Here's how the part is built. I have some questions about the finished solid (model axes, mm). Face numbers are marked on the shaded views. Round coordinates to 2 decimals unless told otherwise and drop trailing zeros. Loops run counter-clockwise (first coordinate to the right, second up) from the corner with the lowest first, then second, coordinate; pieces in that order, holes last. Notation, with made-up numbers: (-0.75, 53.25) - (32.25, 53.25) arc R21 cw to (32.25, 62.25) - close; hole circle Ø4 at (-31.75, -39). An arc over 180 degrees is marked (long way). Answer as a JSON object with one key per item and string values. Group by question number.
1) I want a section at A-A, the plane x = -1. Please give me the cut outline in (y, z) (3 decimals).
2) I want a section at B-B, the plane z = 7.5. Please give me the cut outline in (x, y), then the cut area to 3 significant figures.
3) Will these pins go through, and if not, where does the flat tip stop? P1, Ø4, axis at x = 4.5, z = 3, coming from the -Y side; P2, Ø2, axis at x = -1, y = 13, coming from the -Z side; P3, Ø2, axis at y = 12.5, z = 2.5, coming from the -X side; P4, Ø2.5, axis at x = 0, y = 14.15, coming from the +Z side.
4) If we mould it in two halves opening along X, with no side actions, what happens to the marked faces 1, 2 and 3? For each: pulls with the +X half, pulls with the -X half, needs draft (parallel to the pull), parting line crosses it, or undercut.
5) I want a section at C-C, the plane x = -12. Please give me the cut outline in (y, z) (3 decimals), then the cut area to 3 significant figures.
6) If I drill on line 1 along Y through (x, z) = (10.5, 2.75); line 2 along Y through (x, z) = (5.5, 2.5); line 3 along X through (y, z) = (11, 2.75), over which ranges is the centre line in solid material (lowest first)? Write a range as [from, to].
7) I want a section at D-D, the plane z = 2. Please give me the cut outline in (x, y).
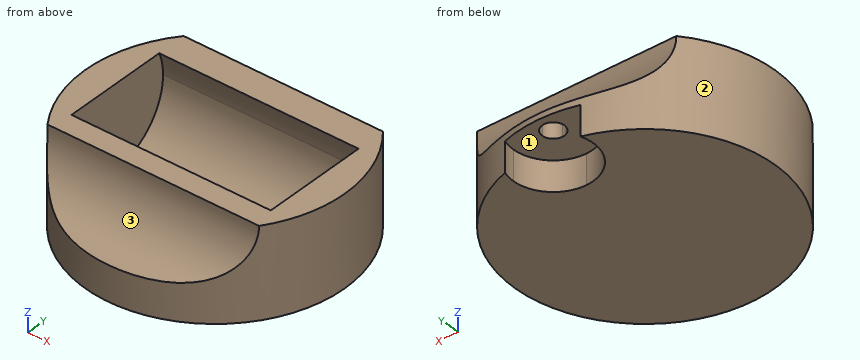
from build123d import *

# Parameters (mm, degrees)
F0_R      = 16.51
F1_DEPTH  = 11.43
F3_DEPTH  = 12.7
F5_DEPTH  = 3.81
F7_DEPTH  = 11.43
F9_DEPTH  = 25.4
F11_DEPTH = 25.4


with BuildPart() as f1:
    # F0 (on Top) → F1 (new body)
    with BuildSketch(Plane.XY):
        Circle(F0_R)
    extrude(amount=F1_DEPTH)

    # F2 (on Right) → F3 (cut, symmetric)
    with BuildSketch(Plane.YZ):
        with BuildLine():
            ThreePointArc((0, 1.162998), (5.208549, 3.32045), (7.366, 8.528998))
            ThreePointArc((7.366, 8.528998), (-5.208549, 13.737547), (0, 1.162998))
        make_face()
    extrude(amount=F3_DEPTH, both=True, mode=Mode.SUBTRACT)

    # F4 (on Top) → F5 (cut)
    with BuildSketch(Plane.XY):
        with BuildLine():
            ThreePointArc((0, 9.0678), (3.592102, 10.555698), (5.08, 14.1478))
            ThreePointArc((5.08, 14.1478), (-3.592102, 17.739902), (0, 9.0678))
        make_face()
    extrude(amount=F5_DEPTH, mode=Mode.SUBTRACT)

    # F6 (on Top) → F7 (cut, through all)
    with BuildSketch(Plane.XY):
        with BuildLine():
            ThreePointArc((0, 12.7508), (0.987828, 13.159972), (1.397, 14.1478))
            ThreePointArc((1.397, 14.1478), (-0.987828, 15.135628), (0, 12.7508))
        make_face()
    extrude(amount=F7_DEPTH, mode=Mode.SUBTRACT)

    # F8 (on Right) → F9 (cut, symmetric)
    with BuildSketch(Plane.YZ):
        with BuildLine():
            ThreePointArc((-16.51, 4.445), (-11.570859, 6.490859), (-9.525, 11.43))
            ThreePointArc((-9.525, 11.43), (-21.449141, 16.369141), (-16.51, 4.445))
        make_face()
    extrude(amount=F9_DEPTH, both=True, mode=Mode.SUBTRACT)

    # F10 (on Right) → F11 (cut, symmetric)
    with BuildSketch(Plane.YZ):
        with BuildLine():
            ThreePointArc((16.51, 4.519911), (22.094443, 6.142438), (24.515244, 11.43))
            ThreePointArc((24.515244, 11.43), (12.966045, 16.717562), (16.51, 4.519911))
        make_face()
    extrude(amount=F11_DEPTH, both=True, mode=Mode.SUBTRACT)


solid = f1.part
Outcome:
{
 "1": {"outline": "(-16.48, 0) - (9.167, 0) - (9.167, 3.81) - (13.172, 3.81) - (13.172, 5.971) arc R6.985 cw to (10.545, 11.43) - (6.771, 11.43) arc R7.366 cw (long way) to (-6.771, 11.43) - (-9.525, 11.43) arc R6.985 cw to (-16.48, 4.445) - close; (15.123, 3.81) - (16.48, 3.81) - (16.48, 4.524) arc R6.985 cw to (15.123, 4.873) - close"},
 "2": {"outline": "(-12.54, -10.74) - (12.54, -10.74) arc R16.51 ccw to (11.59, 11.76) - (-11.59, 11.76) arc R16.51 ccw to start; hole (-12.7, -7.29) - (12.7, -7.29) - (12.7, 7.29) - (-12.7, 7.29) - close", "area": "309 mm^2"},
 "3": {"P1": "y = -16.32", "P2": "z = 3.81", "P3": "x = -11.85", "P4": "through"},
 "4": {"face 1": "undercut", "face 2": "parting line crosses it", "face 3": "needs draft"},
 "5": {"outline": "(-11.339, 0) - (11.339, 0) - (11.339, 8.195) arc R6.985 cw to (10.545, 11.43) - (6.771, 11.43) arc R7.366 cw (long way) to (-6.771, 11.43) - (-9.525, 11.43) arc R6.985 cw to (-11.339, 6.734) - close", "area": "125 mm^2"},
 "6": {"line 1": "[-12.74, -4.57], [4.57, 12.74]", "line 2": "[-15.57, -4.23], [4.23, 15.57]", "line 3": "[-12.31, -3.99], [3.99, 12.31]"},
 "7": {"outline": "(-4.81, 15.8) arc R16.51 ccw (long way) to (4.81, 15.8) arc R5.08 cw to (5.08, 14.15) arc R5.08 cw to (0, 9.07) arc R5.08 cw to start; hole (-12.7, -3.41) - (12.7, -3.41) - (12.7, 3.41) - (-12.7, 3.41) - close"}
}
